Design review of the part built by this model. Coordinates are the model's own, in mm. Coordinates: 2 decimals unless noted, no trailing zeros. Write each loop counter-clockwise with the first axis right and the second up, starting at its lowest first coordinate (ties: lowest second). Pieces come first, ordered by that corner, then holes. Notation, with made-up numbers: (-7, 13.5) - (37, 13.5) arc R25 ccw to (37, 36.5) - close; hole circle Ø2 at (59, 12). An arc over 180 degrees is marked (long way). One line per item, written item: value.
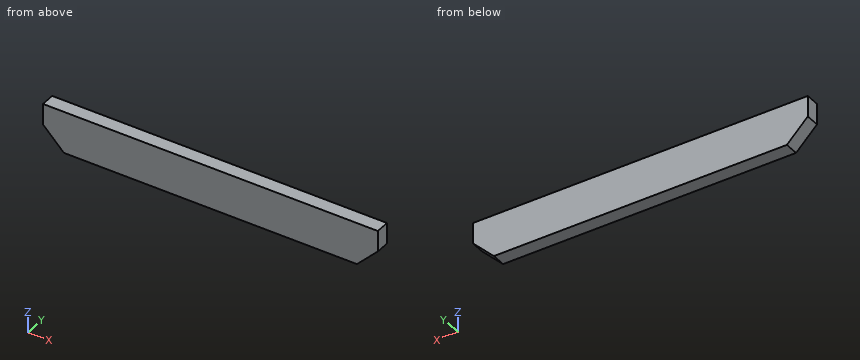
from build123d import *

# Parameters (mm, degrees)
F0_W     = 50
F0_H     = 150
F1_DEPTH = 600
F3_DEPTH = 50.001


# Not quite as in the source:
# - a pattern or mirror of a feature is missing from the dataset's text; its kind, count and spacing are read off the source's solid


with BuildPart() as f1:
    # F0 (on Right) → F1 (new body, symmetric)
    with BuildSketch(Plane.YZ):
        Rectangle(F0_W, F0_H)
    extrude(amount=F1_DEPTH, both=True)

    # F2 (on face) → F3 (cut, through all)
    with BuildSketch(Plane.XZ.offset(25)):
        Polygon((-525, -75), (-600, 0), (-600, -75), align=None)
    f3 = extrude(amount=-F3_DEPTH, mode=Mode.SUBTRACT)

    # F3_copies: F3 across plane
    add(f3.mirror(Plane(origin=(0, 0, 0), x_dir=(0, 0, 1), z_dir=(1, 0, 0))), mode=Mode.SUBTRACT)


solid = f1.part
1. Wall thickness on line 1 along Z through (x, y) = (535.5, 19); line 2 along X through (y, z) = (8, -49); line 3 along X through (y, z) = (20.5, -19.5): over which ranges is each line inside the solid? List them lowest first.
Answer block:
line 1: z = -64.5 to 75
line 2: x = -551 to 551
line 3: x = -580.5 to 580.5
2. Consider section B-B, the plane z = -30. Write out the cut boundary in (x, y).
Answer block:
outline: (-570, -25) - (570, -25) - (570, 25) - (-570, 25) - close
3. Consider section A-A, the plane y = -4. Write out the cut boundary in (x, z), then the cut area to 3 significant figures.
Answer block:
outline: (-600, 0) - (-525, -75) - (525, -75) - (600, 0) - (600, 75) - (-600, 75) - close
area: 174,000 mm^2
4. Insertion check: pin 1 Ø5 at (y, z) = (-17.5, -13) entering from -X. The pin has a flat end and moves straight along its axis. Give the tip position at first contact, or say it passes through.
Answer block:
pin 1: stops at x = -589.5
